Geometry check sheet. Reference: drawing and pictorial views, mm from the part's lowest x, y, z. A direction names the side the tool comes from. Coordinates: 2 decimals unless noted, no trailing zeros. Write each loop counter-clockwise with the first axis right and the second up, starting at its lowest first coordinate (ties: lowest second). Pieces come first, ordered by that corner, then holes. Notation, with made-up numbers: (37.25, 17) -> (73.25, 17) arc R23 ccw to (73.25, 42) -> close; hole circle Ø4 at (79.5, 43). An arc over 180 degrees is marked (long way). Answer in a Markdown table with one row per item.
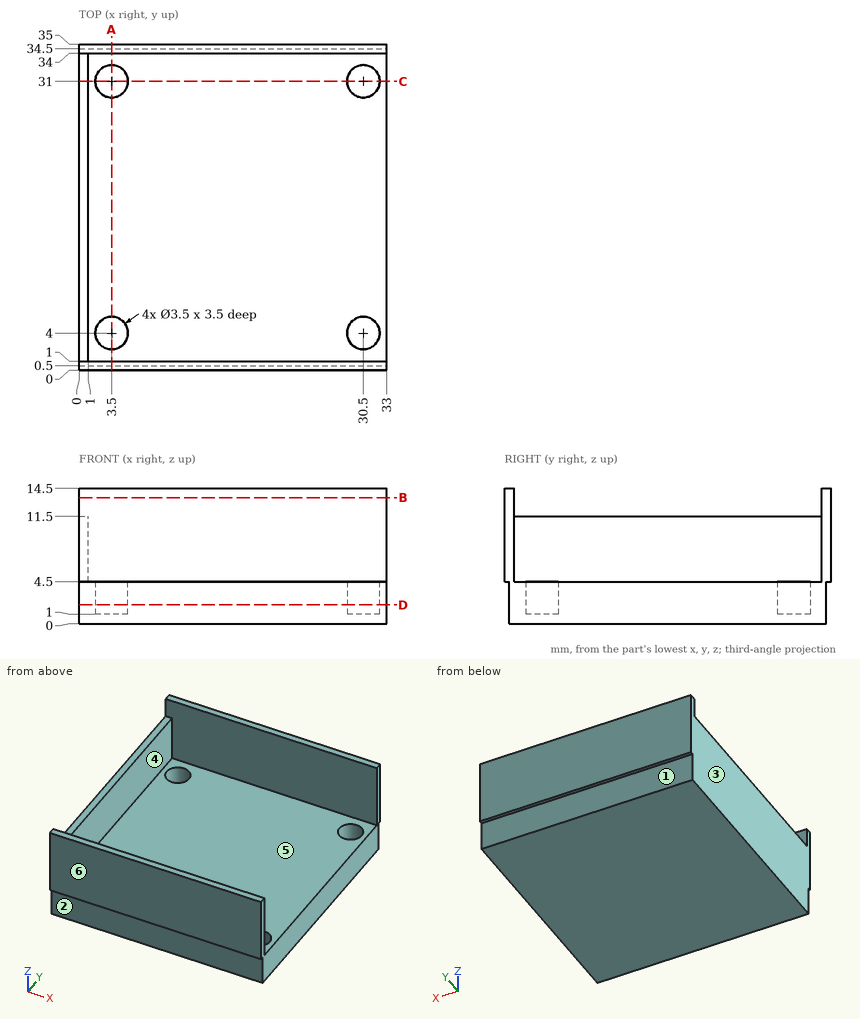
1. Tool access check on the marked faces 5 and 6. Record the directions out of +Z, -Z, +X, -X, +Y, -Y that give a thin tool (end or side, any length) a straight path to the whole face; none if there is none.
Geometry says:
| item | result |
|---|---|
| face 5 | +Z, +X |
| face 6 | +Z, -Z, +X, -X, -Y |
2. Section check C-C, the plane y = 31. Record the boundary of the cut face in (x, z).
Geometry says:
| item | result |
|---|---|
| outline | (0, 0) -> (33, 0) -> (33, 4.5) -> (32.25, 4.5) -> (32.25, 1) -> (28.75, 1) -> (28.75, 4.5) -> (5.25, 4.5) -> (5.25, 1) -> (1.75, 1) -> (1.75, 4.5) -> (1, 4.5) -> (1, 11.5) -> (0, 11.5) -> close |
3. Section check B-B, the plane z = 13.5. Record the boundary of the cut face in (x, y).
Geometry says:
| item | result |
|---|---|
| outline | (0, 0) -> (33, 0) -> (33, 1) -> (0, 1) -> close; (0, 34) -> (33, 34) -> (33, 35) -> (0, 35) -> close |
4. Thickness scan on line 1 (Y direction, x = 3.5, z = 2.2); line 2 (X direction, y = 4, z = 3.6); line 3 (Y direction, x = 28.5, z = 13). Record the ranges inside material, lowest first. Write a range as from..to.
Geometry says:
| item | result |
|---|---|
| line 1 | 0.5..2.25, 5.75..29.25, 32.75..34.5 |
| line 2 | 0..1.75, 5.25..28.75, 32.25..33 |
| line 3 | 0..1, 34..35 |
5. Depth check by flat-ended pin: P1, Ø3.5, axis at y = 12, z = 9.5, coming from the +X side; P2, Ø3, axis at x = 4, y = 3, coming from the +Z side; P3, Ø1.8, axis at x = 30, y = 31.5, coming from the +Z side; P4, Ø2, axis at y = 17, z = 13, coming from the -X side. Enter the tip coordinate at first touch or a pass-through.
Geometry says:
| item | result |
|---|---|
| P1 | x = 1 |
| P2 | z = 4.5 |
| P3 | z = 1 |
| P4 | through |
6. Section check A-A, the plane x = 3.5. Record the boundary of the cut face in (y, z), plus the area to 4 significant figures.
Geometry says:
| item | result |
|---|---|
| outline | (0, 4.5) -> (0.5, 4.5) -> (0.5, 0) -> (34.5, 0) -> (34.5, 4.5) -> (35, 4.5) -> (35, 14.5) -> (34, 14.5) -> (34, 4.5) -> (32.75, 4.5) -> (32.75, 1) -> (29.25, 1) -> (29.25, 4.5) -> (5.75, 4.5) -> (5.75, 1) -> (2.25, 1) -> (2.25, 4.5) -> (1, 4.5) -> (1, 14.5) -> (0, 14.5) -> close |
| area | 148.5 mm^2 |
7. Mould release check, pull along Y, two halves, no side actions. Record for the marked faces 1, 2, 3 and 4: released by +Y, released by -Y, zero draft, split by the parting line, or undercut.
Geometry says:
| item | result |
|---|---|
| face 1 | released by +Y |
| face 2 | released by -Y |
| face 3 | zero draft |
| face 4 | undercut |
8. Section check D-D, the plane z = 2. Record the boundary of the cut face in (x, y).
Geometry says:
| item | result |
|---|---|
| outline | (0, 0.5) -> (33, 0.5) -> (33, 34.5) -> (0, 34.5) -> close; hole circle Ø3.5 at (3.5, 4); hole circle Ø3.5 at (3.5, 31); hole circle Ø3.5 at (30.5, 4); hole circle Ø3.5 at (30.5, 31) |
